Study the drawing (mm; zero at the part's minimum x, y, z) and answer. A direction names the side the tool comes from. Round coordinates to 2 decimals unless told otherwise and drop trailing zeros. Order: outer loops, then holes, each group sorted by start corner. A loop starts at its lowest first (then second) coordinate and runs counter-clockwise, first axis right, second up. Notation, with made-up numbers: M 30,-4 L 86,-4 A25 cw 86,20 Z; hole C 43,48.5 d4. An arc over 180 degrees is marked long. Put each result on its own line as item: value. Start each with the question number.
1. The part is cut by section C-C (x = 49). Give the vertices of the cut face in (y, z).
2. The part is cut by section B-B (z = 38.1). Give the vertices of the cut face in (x, y).
3. Which of the six approach directions +Z, -Z, +X, -X, +Y, -Y give full straight-line access (tool end or side, diameter ignored) to the marked faces 1 and 2?
4. The part is cut by section D-D (y = 29). Give the vertices of the cut face in (x, z), then the cut area to 3 significant figures.
5. The part is cut by section A-A (x = 31.75). Give the vertices of the cut face in (y, z).
6. Each of these flat-tipped pins is pushed along its axis until it touches: pin 1 Ø7.5 at (x, y) = (40, 23.5) entering from +Z; pin 2 Ø12 at (x, y) = (51.5, 11) entering from +Z; pin 3 Ø11.5 at (x, z) = (31.75, 38.1) entering from -Y. Where does it stop, or does it pass through?
7. Consider line 1 (Z direction, x = 31.75, y = 3.75); line 2 (X direction, y = 3, z = 38); line 3 (Y direction, x = 61.5, z = 50). Determine where each line is inside the solid, lowest interval first.
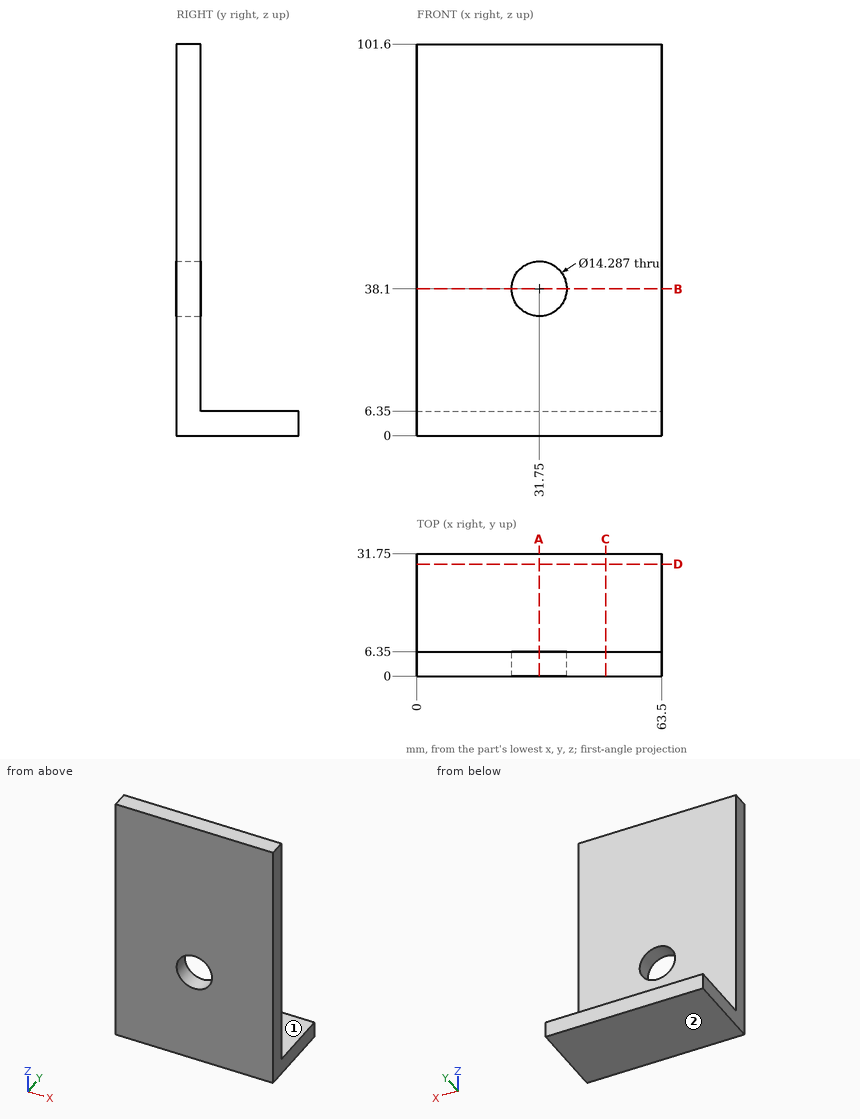
Resolved:
1. outline: M 0,0 L 31.75,0 L 31.75,6.35 L 6.35,6.35 L 6.35,101.6 L 0,101.6 Z
2. outline: M 0,0 L 24.61,0 L 24.61,6.35 L 0,6.35 Z; M 38.89,0 L 63.5,0 L 63.5,6.35 L 38.89,6.35 Z
3. face 1: +Z, +X, -X, +Y
3. face 2: -Z, +X, -X, +Y, -Y
4. outline: M 0,0 L 63.5,0 L 63.5,6.35 L 0,6.35 Z
4. area: 403 mm2
5. outline: M 0,0 L 31.75,0 L 31.75,6.35 L 6.35,6.35 L 6.35,30.96 L 0,30.96 Z; M 0,45.24 L 6.35,45.24 L 6.35,101.6 L 0,101.6 Z
6. pin 1: z = 6.35
6. pin 2: z = 101.6
6. pin 3: through
7. line 1: 0 to 30.96, 45.24 to 101.6
7. line 2: 0 to 24.61, 38.89 to 63.5
7. line 3: 0 to 6.35
